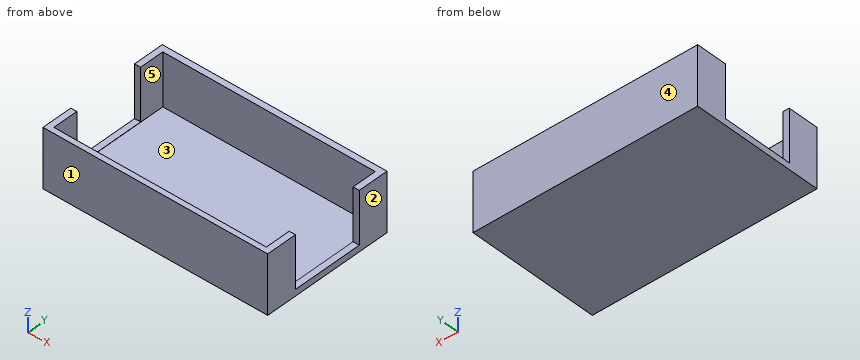
```python
from build123d import *

# Parameters (mm, degrees)
SKETCH_W        = 73
SKETCH_H        = 43
PAD_DEPTH       = 19
SKETCH001_W     = 69.017719
SKETCH001_H     = 39.257344
POCKET_DEPTH    = 17
SKETCH002_W     = 23
SKETCH002_H     = 17
POCKET001_DEPTH = 80


with BuildPart() as part:
    # Sketch → Pad (new body)
    with BuildSketch(Plane.XY):
        with Locations((-36.5, -21.5)):
            Rectangle(SKETCH_W, SKETCH_H)
    extrude(amount=PAD_DEPTH)

    # Sketch001 (on Face6 of Pad) → Pocket (cut)
    with BuildSketch(Plane.XY.offset(19)):
        with Locations((-36.531126, -21.631982)):
            Rectangle(SKETCH001_W, SKETCH001_H)
    extrude(amount=-POCKET_DEPTH, mode=Mode.SUBTRACT)

    # Sketch002 (on Face3 of Pocket) → Pocket001 (cut)
    with BuildSketch(Plane.YZ):
        with Locations((-21.5, 10.579726)):
            Rectangle(SKETCH002_W, SKETCH002_H)
    extrude(amount=-POCKET001_DEPTH, mode=Mode.SUBTRACT)


solid = part.part
```
Input: part model. Units: mm. Frame: model coordinates. Face numbers are marked on the shaded views. A direction names the side the tool comes from. Round coordinates to 2 decimals unless told otherwise and drop trailing zeros. Loops run counter-clockwise (first coordinate to the right, second up) from the corner with the lowest first, then second, coordinate; pieces in that order, holes last. Notation, with made-up numbers: (55, -38) - (88, -38) arc R31 ccw to (88, -6) - close; hole circle Ø8 at (31.25, -29.5). An arc over 180 degrees is marked (long way). One line per item, written item: value. Start each with the question number.
(1) Section A-A, the plane z = 6. Return loops of the section in (x, y), plus the area to 3 significant figures.
(2) Draft query along Y for the marked faces 1, 2 and 3. Return one class per face: +Y half, -Y half, draft (parallel to the pull), parting line (faces both ways), or undercut.
(3) Access query for the marked faces 4 and 5. Directions: +Z, -Z, +X, -X, +Y, -Y. A direction counts if a zero-diameter tool reaches every point of the face in a straight line with its end or side. Return the directions, or none.
(4) Contact query for flat-ended pins moving along their axis: P1, Ø0.6, axis at x = -72, y = -18, coming from the +Z side; P2, Ø6, axis at x = -50.5, y = -22, coming from the +Z side. Output: stop coordinate, or through.
(5) Ray query, line 1 (Y direction, x = -39.5, z = 5.75); line 2 (X direction, y = -5.5, z = 2.25); line 3 (Z direction, x = -42.5, y = -31). Return the intervals inside material, ascending. Write a range as [from, to].
(6) Section B-B, the plane y = -15. Return loops of the section in (x, z), plus the area to 3 significant figures.
(7) Section C-C, the plane x = -48.5. Return loops of the section in (y, z).
Results below:
1. outline: (-73, -43) - (0, -43) - (0, -33) - (-2.02, -33) - (-2.02, -41.26) - (-71.04, -41.26) - (-71.04, -33) - (-73, -33) - close; (-73, -10) - (-71.04, -10) - (-71.04, -2) - (-2.02, -2) - (-2.02, -10) - (0, -10) - (0, 0) - (-73, 0) - close
1. area: 338 mm^2
2. face 1: -Y half
2. face 2: draft
2. face 3: undercut
3. face 4: +Z, -Z, +X, -X, +Y
3. face 5: +Z
4. P1: z = 2.08
4. P2: z = 2
5. line 1: [-43, -41.26], [-2, 0]
5. line 2: [-73, -71.04], [-2.02, 0]
5. line 3: [0, 2]
6. outline: (-73, 0) - (0, 0) - (0, 2.08) - (-2.02, 2.08) - (-2.02, 2) - (-71.04, 2) - (-71.04, 2.08) - (-73, 2.08) - close
6. area: 146 mm^2
7. outline: (-43, 0) - (0, 0) - (0, 19) - (-2, 19) - (-2, 2) - (-41.26, 2) - (-41.26, 19) - (-43, 19) - close
